Work out the finished part from the listing and answer in its coordinate system (mm). Give positions to 0.01 mm unless a question says otherwise; leave off trailing zeros. Write each loop counter-clockwise with the first axis right and the second up, starting at its lowest first coordinate (ties: lowest second). Pieces come first, ordered by that corner, then holes. Notation, with made-up numbers: (21, 37.25) - (70, 37.25) arc R22 cw to (70, 61.25) - close; hole circle Ø9 at (20, 77.25). An arc over 180 degrees is marked (long way). Write item = value, one per line.
from build123d import *

# Parameters (mm, degrees)
SKETCH1_W           = 100
SKETCH1_H           = 100
SKETCH1_R           = 2.5
SKETCH1_W_2         = 70
SKETCH1_H_2         = 5
BOSS_EXTRUDE1_DEPTH = 2
FILLET1_R           = 5
FILLET2_R           = 1.5


with BuildPart() as part:
    # Sketch1 → Boss-Extrude1 (new body)
    with BuildSketch(Plane(origin=(0, 0, 0), x_dir=(1, 0, 0), z_dir=(0, 1, 0))):
        Rectangle(SKETCH1_W, SKETCH1_H)
        with Locations((-40, 40)):
            Circle(SKETCH1_R, mode=Mode.SUBTRACT)
        with Locations((40, 40)):
            Circle(SKETCH1_R, mode=Mode.SUBTRACT)
        with Locations((40, -40)):
            Circle(SKETCH1_R, mode=Mode.SUBTRACT)
        with Locations((-40, -40)):
            Circle(SKETCH1_R, mode=Mode.SUBTRACT)
        with Locations((0, -30)):
            Rectangle(SKETCH1_W_2, SKETCH1_H_2, mode=Mode.SUBTRACT)
        with Locations((0, -20)):
            Rectangle(SKETCH1_W_2, SKETCH1_H_2, mode=Mode.SUBTRACT)
        with Locations((0, -10)):
            Rectangle(SKETCH1_W_2, SKETCH1_H_2, mode=Mode.SUBTRACT)
        Rectangle(SKETCH1_W_2, SKETCH1_H_2, mode=Mode.SUBTRACT)
        with Locations((0, 10)):
            Rectangle(SKETCH1_W_2, SKETCH1_H_2, mode=Mode.SUBTRACT)
        with Locations((0, 20)):
            Rectangle(SKETCH1_W_2, SKETCH1_H_2, mode=Mode.SUBTRACT)
        with Locations((0, 30)):
            Rectangle(SKETCH1_W_2, SKETCH1_H_2, mode=Mode.SUBTRACT)
    extrude(amount=BOSS_EXTRUDE1_DEPTH)

    # Fillet1
    fillet1_edges = [part.edges().sort_by_distance(p)[0] for p in [
        (50, 1, 50),
        (-50, 1, 50),
        (-50, 1, -50),
        (50, 1, -50),
    ]]
    fillet(fillet1_edges, radius=FILLET1_R)

    # Fillet2
    fillet2_edges = [part.edges().sort_by_distance(p)[0] for p in [
        (35, 1, -27.5),
        (35, 1, -32.5),
        (-35, 1, -32.5),
        (-35, 1, -27.5),
        (35, 1, 32.5),
        (35, 1, 27.5),
        (-35, 1, 27.5),
        (-35, 1, 32.5),
        (35, 1, 22.5),
        (35, 1, 17.5),
        (-35, 1, 17.5),
        (-35, 1, 22.5),
        (35, 1, 12.5),
        (35, 1, 7.5),
        (-35, 1, 7.5),
        (-35, 1, 12.5),
        (35, 1, 2.5),
        (35, 1, -2.5),
        (-35, 1, -2.5),
        (-35, 1, 2.5),
        (35, 1, -7.5),
        (35, 1, -12.5),
        (-35, 1, -12.5),
        (-35, 1, -7.5),
        (35, 1, -17.5),
        (35, 1, -22.5),
        (-35, 1, -22.5),
        (-35, 1, -17.5),
    ]]
    fillet(fillet2_edges, radius=FILLET2_R)


solid = part.part
1. Straight lines are drawn through the part: line 1 (X direction, y = 0.85, z = -40); line 2 (X direction, y = 0.5, z = 31). For each, find the intervals that lie inside material, in ascending order.
Solution:
line_1 = -50 to -42.5, -37.5 to 37.5, 42.5 to 50
line_2 = -50 to -35, 35 to 50
2. Find section C-C, the plane x = 22. Give the number of separate pieces and of enclosed holes in the cut face, then the cut area to 3 significant figures.
Solution:
separate_pieces = 8
enclosed_holes = 0
area = 130 mm^2
3. Find section B-B, the plane z = 40. Give the vertices of the cut face in (x, y).
Solution:
outline = (-50, 0) - (-42.5, 0) - (-42.5, 2) - (-50, 2) - close; (-37.5, 0) - (37.5, 0) - (37.5, 2) - (-37.5, 2) - close; (42.5, 0) - (50, 0) - (50, 2) - (42.5, 2) - close
4. For a pull along Z with two mould halves and no side action, classify faces 1 (the cylindrical face through (-37.69, 0.99, 40.96)), 2 (the flat face through (-1, 2, -23)), 3 (the cylindrical face through (-49, 1, 48)), 4 (the cylindrical face through (48, 1, -49)) as pulls with the +Z half, pulls with the -Z half, needs draft (parallel to the pull), parting line crosses it, or undercut.
Solution:
face_1 = undercut
face_2 = needs draft
face_3 = pulls with the +Z half
face_4 = pulls with the -Z half
5. Given pin 1 (6 mm diameter, centred on x = -30.5, z = -18, fed in from +Y), flat-ended and moving along its own axis, determine where the tip first touches the part or whether it passes through.
Solution:
pin_1 = 2
6. Find section A-A, the plane x = -40. Give the vertices of the cut face in (y, z), then the cut area to 3 significant figures.
Solution:
outline = (0, -50) - (2, -50) - (2, -42.5) - (0, -42.5) - close; (0, -37.5) - (2, -37.5) - (2, 37.5) - (0, 37.5) - close; (0, 42.5) - (2, 42.5) - (2, 50) - (0, 50) - close
area = 180 mm^2
